Build history of the part. All positions in model axes, mm. A direction names the side the tool comes from. Give positions to 0.01 mm unless a question says otherwise; leave off trailing zeros. Order: outer loops, then holes, each group sorted by start corner. A loop starts at its lowest first (then second) coordinate and runs counter-clockwise, first axis right, second up. Notation, with made-up numbers: M 56,38.25 L 101,38.25 A12 cw 101,53.25 Z; hole C 31,-17.75 d9. An arc over 180 degrees is marked long. Answer as CSV lines item,"result".
from build123d import *

# Parameters (mm, degrees)
SKETCH1_W           = 74
SKETCH1_H           = 8.5
BOSS_EXTRUDE1_DEPTH = 6.5
SKETCH2_W           = 4
SKETCH2_H           = 35
CUT_EXTRUDE1_DEPTH  = 3
SKETCH3_W           = 2.242776622
SKETCH3_H           = 2.782449956
BOSS_EXTRUDE2_DEPTH = 10
BOSS_EXTRUDE3_DEPTH = 1.12
BOSS_EXTRUDE5_START = 1.12
BOSS_EXTRUDE5_DEPTH = 1.12


with BuildPart() as part:
    # Sketch1 → Boss-Extrude1 (new body)
    with BuildSketch(Plane(origin=(0, 0, 0), x_dir=(0, 1, 0), z_dir=(0, 0, 1))):
        Rectangle(SKETCH1_W, SKETCH1_H)
    extrude(amount=BOSS_EXTRUDE1_DEPTH)

    # Sketch2 → Cut-Extrude1 (cut)
    with BuildSketch(Plane.XY.offset(6.5)):
        Rectangle(SKETCH2_W, SKETCH2_H)
    extrude(amount=-CUT_EXTRUDE1_DEPTH, mode=Mode.SUBTRACT)

    # Sketch3 → Boss-Extrude2 (add)
    with BuildSketch(Plane.XY.offset(3.5)):
        Rectangle(SKETCH3_W, SKETCH3_H)
    extrude(amount=BOSS_EXTRUDE2_DEPTH)

    # Sketch4 → Boss-Extrude3 (add)
    with BuildSketch(Plane.YZ):
        with BuildLine():
            Line((-3.093095713, 13.5), (3.093095713, 13.5))
            ThreePointArc((3.093095713, 13.5), (0, 16.593095713), (-3.093095713, 13.5))
        make_face()
    extrude(amount=BOSS_EXTRUDE3_DEPTH)

    # Sketch10 → Boss-Extrude5 (add)
    with BuildSketch(Plane(origin=(0, 0, 0), x_dir=(0, -1, 0), z_dir=(-1, 0, 0)).offset(BOSS_EXTRUDE5_START)):
        with BuildLine():
            Line((3.093095713, 13.5), (-3.093095713, 13.5))
            ThreePointArc((-3.093095713, 13.5), (0, 16.593095713), (3.093095713, 13.5))
        make_face()
    extrude(amount=-BOSS_EXTRUDE5_DEPTH)


solid = part.part
Item 1: Band-saw the part on B-B (x = 0.5). Give the cut face in (y, z), and give its area (3 significant figures).
Geometry says:
outline,"M -37,0 L 37,0 L 37,6.5 L 17.5,6.5 L 17.5,3.5 L 1.39,3.5 L 1.39,13.5 L 3.09,13.5 A3.09 ccw -3.09,13.5 L -1.39,13.5 L -1.39,3.5 L -17.5,3.5 L -17.5,6.5 L -37,6.5 Z"
area,"419 mm2"
Item 2: Pull direction Z, two halves, no side cores. Call faces 4 (the flat face through (0, 1.391, 8)), 5 (the cylindrical face through (-0.016, 0.068, 16.592)), 6 (the flat face through (0, -17.5, 5)): released by +Z, released by -Z, zero draft, split by the parting line, or undercut.
Geometry says:
face 4,"undercut"
face 5,"released by +Z"
face 6,"zero draft"
Item 3: Band-saw the part on D-D (z = 11.25). Give the cut face in (x, y), and give its area (3 significant figures).
Geometry says:
outline,"M -1.12,-1.39 L 1.12,-1.39 L 1.12,1.39 L -1.12,1.39 Z"
area,"6.24 mm2"
Item 4: Drop flat-ended pins along their axis: pin 1 (4.5 mm diameter, centred on x = 1, y = 7, fed in from +Z); pin 2 (1.5 mm diameter, centred on y = -1.5, z = 15, fed in from -X); pin 3 (2.5 mm diameter, centred on x = -0.5, z = 11, fed in from -Y). Give the stop position or say it passes through.
Geometry says:
pin 1,"stops at z = 6.5"
pin 2,"stops at x = -1.12"
pin 3,"stops at y = -1.39"
Item 5: Probe line 1 along Y through (x, z) = (0.5, 3.75); line 2 along Y through (x, z) = (1, 13); line 3 along Z through (x, y) = (1, -10). List the from-to ranges inside material, lowest first. Write a range as from..to.
Geometry says:
line 1,"y = -37..-17.5, -1.39..1.39, 17.5..37"
line 2,"y = -1.39..1.39"
line 3,"z = 0..3.5"
Item 6: Band-saw the part on A-A (z = 5.5). Give the cut face in (x, y), and give its area (3 significant figures).
Geometry says:
outline,"M -4.25,-37 L 4.25,-37 L 4.25,37 L -4.25,37 Z; M -1.12,-1.39 L 1.12,-1.39 L 1.12,1.39 L -1.12,1.39 Z; hole M -2,-17.5 L 2,-17.5 L 2,17.5 L -2,17.5 Z"
area,"495 mm2"
Item 7: 3-axis set-ups, long thin cutter, end or side, ignore diameter. For faces 1 (the flat face through (-1.12, 0, 15)), 2 (the flat face through (0, 2, 13.5)), 3 (the flat face through (2, 0, 5)): which of +Z, -Z, +X, -X, +Y, -Y reach the whole face in a straight line?
Geometry says:
face 1,"+Z, -X, +Y, -Y"
face 2,"+X, -X, +Y"
face 3,"+Z"
